The listing builds one solid part. Answer for the finished solid, in the listing's coordinates (mm). Face numbers are marked on the shaded views. A direction names the side the tool comes from. Round coordinates to 2 decimals unless told otherwise and drop trailing zeros. Write each loop counter-clockwise with the first axis right and the second up, starting at its lowest first coordinate (ties: lowest second). Pieces come first, ordered by that corner, then holes. Notation, with made-up numbers: M -1.75,86 L 17.25,86 A30 ccw 17.25,115 Z; hole C 64.25,17 d8. An arc over 180 degrees is marked long. Write each question's results on one line, items separated by ' | '.
from build123d import *

# Parameters (mm, degrees)
SKETCH1_W           = 18.8
SKETCH1_H           = 20
BOSS_EXTRUDE1_DEPTH = 8
SKETCH2_R           = 1.25
CUT_EXTRUDE1_DEPTH  = 7
SKETCH3_W           = 18.8
SKETCH3_H           = 10
CUT_EXTRUDE2_DEPTH  = 0.5
SKETCH4_W           = 9
SKETCH4_H           = 4.5
CUT_EXTRUDE3_DEPTH  = 20
BOSS_EXTRUDE2_DEPTH = 4
LPATTERN1_COUNT     = 2
LPATTERN1_PITCH     = 22.8
BOSS_EXTRUDE3_DEPTH = 1
LPATTERN3_COUNT     = 2
LPATTERN3_PITCH     = 27.8
SKETCH8_R           = 1.5
BOSS_EXTRUDE4_DEPTH = 0.5
LPATTERN4_COUNT     = 2
LPATTERN4_PITCH     = 29.3


with BuildPart() as part:
    # Sketch1 → Boss-Extrude1 (new body)
    with BuildSketch(Plane(origin=(0, 0, 0), x_dir=(1, 0, 0), z_dir=(0, 1, 0))):
        with Locations((9.4, 10)):
            Rectangle(SKETCH1_W, SKETCH1_H)
    extrude(amount=BOSS_EXTRUDE1_DEPTH)

    # Sketch2 → Cut-Extrude1 (cut)
    with BuildSketch(Plane(origin=(0, 8, 0), x_dir=(1, 0, 0), z_dir=(0, 1, 0))):
        with Locations(Location((4.4, 2.5, 0), (0, 0, 270))):
            Circle(SKETCH2_R)
        with Locations(Location((14.4, 2.5, 0), (0, 0, 270))):
            Circle(SKETCH2_R)
        with Locations(Location((14.4, 17.5, 0), (0, 0, 270))):
            Circle(SKETCH2_R)
        with Locations(Location((4.4, 17.5, 0), (0, 0, 270))):
            Circle(SKETCH2_R)
    extrude(amount=-CUT_EXTRUDE1_DEPTH, mode=Mode.SUBTRACT)

    # Sketch3 → Cut-Extrude2 (cut)
    with BuildSketch(Plane(origin=(0, 8, 0), x_dir=(1, 0, 0), z_dir=(0, 1, 0))):
        with Locations((9.4, 10)):
            Rectangle(SKETCH3_W, SKETCH3_H)
    extrude(amount=-CUT_EXTRUDE2_DEPTH, mode=Mode.SUBTRACT)

    # Sketch4 → Cut-Extrude3 (cut)
    with BuildSketch(Plane(origin=(18.8, 0, 0), x_dir=(0, 0, -1), z_dir=(1, 0, 0))):
        with Locations((10, 2.25)):
            Rectangle(SKETCH4_W, SKETCH4_H)
    extrude(amount=-CUT_EXTRUDE3_DEPTH, mode=Mode.SUBTRACT)

    # Sketch5 → Boss-Extrude2 (add)
    with BuildSketch(Plane(origin=(18.8, 0, 0), x_dir=(0, 0, -1), z_dir=(1, 0, 0))):
        Polygon((5.5, 0), (0.15, 0), (0.15, 7.5), (5.5, 7.5), (14.5, 7.5), (19.85, 7.5), (19.85, 0), (14.5, 0), (14.5, 4.5), (5.5, 4.5), align=None)
    boss_extrude2 = extrude(amount=BOSS_EXTRUDE2_DEPTH)

    # LPattern1: Boss-Extrude2 ×2
    with Locations(*[(-i * LPATTERN1_PITCH, 0, 0) for i in range(1, LPATTERN1_COUNT)]):
        add(boss_extrude2)

    # Sketch6 → Boss-Extrude3 (add)
    with BuildSketch(Plane(origin=(22.8, 0, 0), x_dir=(0, 0, -1), z_dir=(1, 0, 0))):
        Polygon((0, 0), (5, 0), (5.5, 0), (5.5, 4.5), (14.5, 4.5), (14.5, 0), (15, 0), (20, 0), (20, 8), (15, 8), (5, 8), (0, 8), align=None)
    boss_extrude3 = extrude(amount=BOSS_EXTRUDE3_DEPTH)

    # LPattern3: Boss-Extrude3 ×2
    with Locations(*[(-i * LPATTERN3_PITCH, 0, 0) for i in range(1, LPATTERN3_COUNT)]):
        add(boss_extrude3)

    # Sketch8 → Boss-Extrude4 (add)
    with BuildSketch(Plane(origin=(23.8, 0, 0), x_dir=(0, 0, -1), z_dir=(1, 0, 0))):
        with Locations(Location((5, 6.2, 0), (0, 0, 180))):
            Circle(SKETCH8_R)
        with Locations(Location((15, 6.2, 0), (0, 0, 180))):
            Circle(SKETCH8_R)
    boss_extrude4 = extrude(amount=BOSS_EXTRUDE4_DEPTH)

    # LPattern4: Boss-Extrude4 ×2
    with Locations(*[(-i * LPATTERN4_PITCH, 0, 0) for i in range(1, LPATTERN4_COUNT)]):
        add(boss_extrude4)


solid = part.part
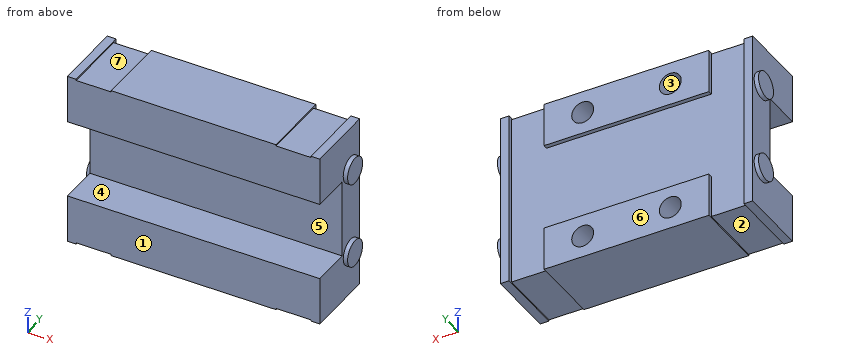
1) A tool of negligible diameter and unlimited length cuts with its end or side. For the marked faces 1, 2, 3 and 4, from which of +Z, -Z, +X, -X, +Y, -Y can it reach the whole face along a straight path? Write none if from no direction.
Return value:
face 1: +Z, -Z, +X, -X, -Y | face 2: -Z, +Y, -Y | face 3: +Y | face 4: +X, -X, -Y
2) Section A-A (y = 3.25) is taken. Determine the outline of the cut face in (x, z).
Return value:
outline: M -5,-20 L -4,-20 L -4,-19.85 L 0,-19.85 L 0,-20 L 18.8,-20 L 18.8,-19.85 L 22.8,-19.85 L 22.8,-20 L 23.8,-20 L 23.8,-14.5 L -5,-14.5 Z; M -5,-5.5 L 23.8,-5.5 L 23.8,0 L 22.8,0 L 22.8,-0.15 L 18.8,-0.15 L 18.8,0 L 0,0 L 0,-0.15 L -4,-0.15 L -4,0 L -5,0 Z; hole C 4.4,-17.5 d2.5; hole C 4.4,-2.5 d2.5; hole C 14.4,-17.5 d2.5; hole C 14.4,-2.5 d2.5
3) Section D-D (x = -0.75) is taken. Determine the outline of the cut face in (y, z).
Return value:
outline: M 0,-19.85 L 7.5,-19.85 L 7.5,-0.15 L 0,-0.15 L 0,-5.5 L 4.5,-5.5 L 4.5,-14.5 L 0,-14.5 Z
4) Section C-C (z = -12.25) is taken. Determine the outline of the cut face in (x, y), then the cut area to 3 significant figures.
Return value:
outline: M -5,4.5 L 23.8,4.5 L 23.8,8 L 22.8,8 L 22.8,7.5 L -4,7.5 L -4,8 L -5,8 Z | area: 87.4 mm²
5) Section B-B (x = 4.4) is taken. Determine the outline of the cut face in (y, z).
Return value:
outline: M 0,-20 L 8,-20 L 8,-18.75 L 1,-18.75 L 1,-16.25 L 8,-16.25 L 8,-15 L 7.5,-15 L 7.5,-5 L 8,-5 L 8,-3.75 L 1,-3.75 L 1,-1.25 L 8,-1.25 L 8,0 L 0,0 L 0,-5.5 L 4.5,-5.5 L 4.5,-14.5 L 0,-14.5 Z
6) Find the intervals of material crossed by line 1 (X direction, y = 6, z = -2.5); line 2 (Z direction, x = 18.25, y = 2); line 3 (Y direction, x = 3, z = -12.75), in increasing order.
Return value:
line 1: -5 to 3.15, 5.65 to 13.15, 15.65 to 23.8 | line 2: -20 to -14.5, -5.5 to 0 | line 3: 4.5 to 7.5
7) The mould has two halves that part along Z. Classify the marked faces 5, 6 and 7: +Z half, -Z half, draft (parallel to the pull), parting line (faces both ways), or undercut.
Return value:
face 5: undercut | face 6: draft | face 7: +Z half
8) Each of these flat-tipped pins is pushed along its axis until it touches: pin 1 (4.5 mm diameter, centred on x = 21.5, y = 5, fed in from -Z); pin 2 (1.2 mm diameter, centred on x = -2.5, y = 2.5, fed in from +Z); pin 3 (1 mm diameter, centred on x = 10, z = -8.5, fed in from -Y); pin 4 (1.2 mm diameter, centred on x = 4.5, z = -2.5, fed in from +Y). Where does it stop, or does it pass through?
Return value:
pin 1: z = -20 | pin 2: z = -0.15 | pin 3: y = 4.5 | pin 4: y = 1
